Here's how the part is built. I have some questions about the finished solid (model axes, mm). Face numbers are marked on the shaded views. A direction names the side the tool comes from. Give positions to 0.01 mm unless a question says otherwise; leave off trailing zeros. Write each loop counter-clockwise with the first axis right and the second up, starting at its lowest first coordinate (ties: lowest second). Pieces come first, ordered by that corner, then holes. Notation, with made-up numbers: (0, -23) -> (55, -23) arc R31 ccw to (55, 14) -> close; hole circle Ø1 at (-2, -6). An arc over 180 degrees is marked (long way). Put each result on its own line as item: value. Start each with the question number.
Autodesk Inventor part; units mm, degrees
ref_plane "YZ Plane" through (0, 0, 0) normal (1, 0, 0) x (0, 1, 0)
ref_plane "XZ Plane" through (0, 0, 0) normal (0, 1, 0) x (-1, 0, 0)
ref_plane "XY Plane" through (0, 0, 0) normal (0, 0, 1) x (1, 0, 0)
sketch "Sketch1" plane through (0, 0, 0) normal (1, 0, 0) x (0, 1, 0)
  line L0 (0, 0) -> (0, -5)
  line L1 (0, -5) -> (17, -5)
  line L2 (17, -5) -> (17, -15)
  line L3 (17, -15) -> (0, -15)
  line L4 (0, -61) -> (33, -61)
  line L5 (33, -61) -> (33, 0)
  line L6 (33, 0) -> (0, 0)
  circle A0 centre (1, -35) radius 3
  arc A1 (0, -29.0839) -> (0, -40.9161) centre (1, -35) ccw
  line L7 (0, -15) -> (0, -29.0839)
  line L8 (0, -61) -> (0, -40.9161)
  dimension "d0" = 5
  dimension "d1" = 17
  dimension "d2" = 10
  dimension "d4" = 33
  dimension "d6" = 6
  dimension "d7" = 1
  dimension "d8" = 20
  dimension "d9" = 6
  dimension "d47" = 46
extrude "Extrusion1" add sketch "Sketch1" along normal blind 25
sketch "Sketch2" plane through (0, 0, 0) normal (-1, 0, 0) x (0, 0, 1)
  line L0 (-70, -8) -> (-20, -8)
  line L1 (-20, -8) -> (-20, 42)
  line L2 (-20, 42) -> (-70, 42)
  line L3 (-70, 42) -> (-70, -8)
  point P0 (0, 0)
  dimension "d12" = 20
  dimension "d13" = 8
  dimension "d14" = 50
  dimension "d15" = 50
extrude "Extrusion2" cut sketch "Sketch2" against normal blind 5
sketch "Sketch3" plane through (5, 0, 0) normal (-1, 0, 0) x (0, 0, 1)
  line L0 (-61, 22) -> (-40, 22)
  line L1 (-40, 22) -> (-40, 30)
  line L2 (-40, 30) -> (-61, 30)
  line L3 (-61, 30) -> (-61, 22)
  line L4 (-61, 11) -> (-40, 11)
  line L5 (-40, 11) -> (-40, 19)
  line L6 (-40, 19) -> (-61, 19)
  line L7 (-61, 19) -> (-61, 11)
  line L8 (-61, 33) -> (-20, 33)
  point P0 (0, 0)
  dimension "d18" = 8
  dimension "d19" = 8
  dimension "d20" = 21
  dimension "d21" = 3
  dimension "d22" = 3
extrude "Extrusion3" cut sketch "Sketch3" against normal up to next
sketch "Sketch4" plane through (0, 33, 0) normal (0, 1, 0) x (1, 0, 0)
  circle A0 centre (15, 53) radius 4.1
  line L0 (5, 61) -> (25, 61)
  point P0 (0, 0)
  point P1 (15, 61)
  dimension "d25" = 8.2
  dimension "d26" = 8
extrude "Extrusion4" cut sketch "Sketch4" against normal through all
sketch "Sketch5" plane through (5, 11, -40) normal (0, 1, 0) x (1, 0, 0)
  circle A0 centre (10, 13) radius 4.1
  circle A1 centre (10, 13) radius 5
  point P0 (-5, -40)
  dimension "d29" = 10
extrude "Extrusion5" add sketch "Sketch5" along normal blind 0.5
pattern_linear "Rectangular Pattern1" count 2 spacing 11 along (0, 1, 0) of "Extrusion5"
pattern_linear "Rectangular Pattern2" count 2 spacing 7.5 along (0, 1, 0) of "Extrusion5", "Rectangular Pattern1"
sketch "Sketch6" plane through (25, 0, 0) normal (1, 0, 0) x (0, 0, -1)
  circle A0 centre (27, 20) radius 6
  line L0 (61, 33) -> (0, 33)
  line L1 (0, 33) -> (0, 0)
  dimension "d38" = 12
  dimension "d39" = 13
  dimension "d40" = 27
extrude "Extrusion6" cut sketch "Sketch6" against normal up to surface (20 mm away)
fillet "Fillet1" radius 3 6 edges at (25, 31.5, -61) (25, 20.5, -61) (25, 5.5, -61) (5, 31.5, -61) (5, 20.5, -61) (5, 5.5, -61)
fillet "Fillet2" radius 10 1 edges at (12.5, 33, 0)
sketch "Sketch7" plane through (0, 33, -20) normal (0, 1, 0) x (1, 0, 0)
  spline S0 degree 2 poles (15.5392, -0.9329) (15.5392, -1.06) (15.5119, -1.3597) knots 0 0 0 1 1 1
  spline S1 degree 2 poles (15.5119, -1.3597) (15.4847, -1.6684) (15.4847, -1.8137) knots 0 0 0 1 1 1
  spline S2 degree 2 poles (15.4847, -1.8137) (15.4847, -3.2393) (15.9115, -4.5742) knots 0 0 0 1 1 1
  spline S3 degree 2 poles (15.9115, -4.5742) (16.084, -5.1281) (16.084, -5.3642) knots 0 0 0 1 1 1
  spline S4 degree 2 poles (16.084, -5.3642) (16.084, -5.682) (15.5846, -6.0362) (15.3576, -6.0362) knots 0 0 0 1 2 2 2
  spline S5 degree 2 poles (15.3576, -6.0362) (15.2577, -6.0362) (14.8763, -5.9454) knots 0 0 0 1 1 1
  spline S6 degree 2 poles (14.8763, -5.9454) (14.395, -5.8273) (13.7866, -5.7547) knots 0 0 0 1 1 1
  line L0 (13.7866, -5.7547) -> (9.4643, -5.2825)
  spline S7 degree 2 poles (9.4643, -5.2825) (8.8468, -5.228) (8.4836, -5.1372) (8.193, -4.774) (8.193, -4.4561) knots 0 0 0 1 2 3 3 3
  spline S8 degree 2 poles (8.193, -4.4561) (8.193, -4.211) (8.5653, -3.8296) (8.7832, -3.8296) knots 0 0 0 1 2 2 2
  spline S9 degree 2 poles (8.7832, -3.8296) (8.983, -3.8296) (9.4915, -3.9295) knots 0 0 0 1 1 1
  spline S10 degree 2 poles (9.4915, -3.9295) (10.227, -4.0657) (14.3678, -4.556) (14.4949, -4.556) knots 0 0 0 1 2 2 2
  spline S11 degree 2 poles (14.4949, -4.556) (14.6402, -4.556) (14.6402, -4.5015) knots 0 0 0 1 1 1
  spline S12 degree 2 poles (14.6402, -4.5015) (14.6402, -4.3018) (14.504, -3.4119) knots 0 0 0 1 1 1
  spline S13 degree 2 poles (14.504, -3.4119) (14.4313, -2.9942) (14.4132, -2.5674) knots 0 0 0 1 1 1
  spline S14 degree 2 poles (14.4132, -2.5674) (14.3587, -1.3506) (14.2316, -0.8602) knots 0 0 0 1 1 1
  spline S15 degree 2 poles (14.2316, -0.8602) (14.1952, -0.7059) (14.1952, -0.6332) knots 0 0 0 1 1 1
  spline S16 degree 2 poles (14.1952, -0.6332) (14.1952, -0.3426) (14.5403, -0.0157) (14.7764, -0.0157) knots 0 0 0 1 2 2 2
  spline S17 degree 2 poles (14.7764, -0.0157) (15.1215, -0.0157) (15.5392, -0.5787) (15.5392, -0.9329) knots 0 0 0 1 2 2 2
  point P0 (0, -20)
  point P1 (8.193, -6.6991)
extrude "Extrusion7" add sketch "Sketch7" along normal blind 0.5
sketch "Sketch8" plane through (0, 0, 0) normal (0, 0, 1) x (1, 0, 0)
  circle A0 centre (5, 5) radius 2.1
  circle A1 centre (21, 5) radius 2.1
  line L0 (0, 0) -> (25, 0)
  line L1 (25, 23) -> (25, 0)
  line L2 (0, 23) -> (0, 0)
  dimension "d48" = 4.2
  dimension "d49" = 5
  dimension "d50" = 4
  dimension "d51" = 5
extrude "Extrusion8" cut sketch "Sketch8" against normal up to next
equation "\"d18\" = d19"
equation "\"d21\" = d22"
properties material "ABS Plastic"
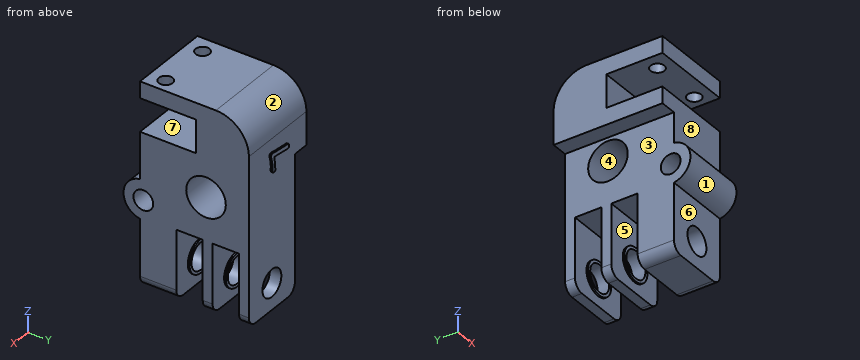
1) Which directions (+Z, -Z, +X, -X, +Y, -Y) give clear straight access to the entire face, cutting with the end or side of a thin tool? Please do the marked faces 5, 6, 7 and 8.
2) I'm going to push flat-ended pins straight in: pin 1 Ø3 at (x, z) = (18.5, -22.5) entering from +Y; pin 2 Ø8 at (x, z) = (17, -52.5) entering from -Y; pin 3 Ø5 at (y, z) = (9, -31.5) entering from -X; pin 4 Ø5 at (y, z) = (1, -35) entering from +X (1 decimal). Where does each tip first touch, or does it pass through?
3) I need wall thicknesses on probe 1 along Z at (x, y) = (10.75, 1); probe 2 along Y at (x, z) = (13.75, -44); probe 3 along Y at (x, z) = (17, -35). Which ranges of each line are inside material? Lowest first, please.
4) I want a section at A-A, the plane y = 1. Write out the boundary of the cut face in (x, z), and give its area (3 significant figures).
5) Thinking about a two-plate mould opening in Y: for the marked faces 1, 2, 3 and 4, which applies, released by +Y, released by -Y, zero draft, split by the parting line, or undercut?
6) I want a section at C-C, the plane z = -27. Write out the boundary of the cut face in (x, y).
7) I want a section at D-D, the plane x = 6. Write out the boundary of the cut face in (y, z).
8) I want a section at B-B, the plane y = 10. Write out the boundary of the cut face in (x, z), and give its area (3 significant figures).
Established:
1. face 5: none
1. face 6: -Z, +X, -X, -Y
1. face 7: +X, -X, -Y
1. face 8: +Z, +X, -X, -Y
2. pin 1: stops at y = 33
2. pin 2: stops at y = 0
2. pin 3: stops at x = 5
2. pin 4: passes through
3. probe 1: z = -61 to -38, -32 to -15, -5 to 0
3. probe 2: y = 0 to 11, 19 to 22, 30 to 33
3. probe 3: y = -5 to -2, 4 to 33
4. outline: (0, -20) -> (5, -20) -> (5, -32) -> (25, -32) -> (25, -15) -> (0, -15) -> close; (0, -5) -> (25, -5) -> (25, 0) -> (0, 0) -> close; (5, -58) arc R3 ccw to (8, -61) -> (22, -61) arc R3 ccw to (25, -58) -> (25, -38) -> (5, -38) -> close; hole circle Ø8.2 at (15, -53)
4. area: 893 mm2
5. face 1: released by -Y
5. face 2: released by +Y
5. face 3: zero draft
5. face 4: undercut
6. outline: (5, 0) -> (25, 0) -> (25, 14) -> (5, 14) -> close; (5, 26) -> (25, 26) -> (25, 33) -> (5, 33) -> close
7. outline: (0, -60.24) -> (11, -60.24) -> (11, -40) -> (19, -40) -> (19, -60.24) -> (22, -60.24) -> (22, -40) -> (30, -40) -> (30, -60.24) -> (33, -60.24) -> (33, -10) arc R10 ccw to (23, 0) -> (6.85, 0) -> (6.85, -5) -> (17, -5) -> (17, -15) -> (0, -15) -> (0, -29.08) arc R6 ccw to (0, -40.92) -> close; (0, -5) -> (3.15, -5) -> (3.15, 0) -> (0, 0) -> close; hole circle Ø6 at (1, -35); hole circle Ø12 at (20, -27)
8. outline: (0, -20) -> (5, -20) -> (5, -58) arc R3 ccw to (8, -61) -> (22, -61) arc R3 ccw to (25, -58) -> (25, -15) -> (0, -15) -> close; (0, -5) -> (25, -5) -> (25, 0) -> (0, 0) -> close; hole circle Ø8.2 at (15, -53)
8. area: 1,010 mm2
